The model under review builds one solid part; all positions refer to its coordinate system, in mm. A direction names the side the tool comes from. Coordinates: 2 decimals unless noted, no trailing zeros. Write each loop counter-clockwise with the first axis right and the second up, starting at its lowest first coordinate (ties: lowest second). Pieces come first, ordered by that corner, then holes.
1) Add section B-B, the plane z = 2.25. State the section outline as (x, y) points, then the cut area to 3 significant figures.
2) For line 1 (X direction, y = 0.2, z = -5.5); line 2 (X direction, y = 0.95, z = 2.75); line 3 (Y direction, x = 1.25, z = -3.75), list the stretches that pass through material, from the lowest coordinate up.
3) For P1, Ø0.9, axis at x = -0.5, y = -0.5, coming from the +Z side, flat-tipped, find the tip position at first contact; note if it passes through.
4) Machinability: for faces 3 (the cylindrical face through (-1.5, 0.07, 0)), 4 (the flat face through (-0.4, -0.4, -0.456)), which of the approach directions +Z, -Z, +X, -X, +Y, -Y give a long, thin tool a straight path to every point of the face, cutting with its end or side? Answer none if there is none.
5) Add section A-A, the plane y = 0.9. Give the number of separate pieces and of enclosed holes in the cut face, then the cut area to 3 significant figures.
6) Mouldability with a two-part tool opening along Z and no side actions: class faces 1 (the flat face through (-0.4, -0.4, -2.589)), 2 (the cylindrical face through (-1.5, 0.07, 2.14)) as released by +Z, released by -Z, zero draft, split by the parting line, or undercut.
from build123d import *

# Parameters (mm, degrees)
SKETCH1_R               = 1.5
BOSS_EXTRUDE1_DEPTH     = 4.8
SKETCH2_W               = 0.2
SKETCH2_H               = 3
CUT_EXTRUDE1_DEPTH      = 2.5
CUT_EXTRUDE1_DEPTH_BACK = 2.5
SKETCH3_R               = 0.375
BOSS_EXTRUDE2_DEPTH     = 6.5
SKETCH4_RX              = 0.5
SKETCH4_RY              = 0.25
BOSS_EXTRUDE3_DEPTH     = 1


with BuildPart() as part:
    # Sketch1 → Boss-Extrude1 (new body, symmetric)
    with BuildSketch(Plane.XY):
        Circle(SKETCH1_R)
    extrude(amount=BOSS_EXTRUDE1_DEPTH, both=True)

    # Sketch2 → Cut-Extrude1 (cut, two sides)
    with BuildSketch(Plane(origin=(0, 0, 0), x_dir=(0, 0, -1), z_dir=(1, 0, 0))) as cut_extrude1_sk:
        with Locations((-3.2, 0)):
            Rectangle(SKETCH2_W, SKETCH2_H)
        with Locations((-2.488888889, 0)):
            Rectangle(SKETCH2_W, SKETCH2_H)
        with Locations((-1.777777778, 0)):
            Rectangle(SKETCH2_W, SKETCH2_H)
        with Locations((-1.066666667, 0)):
            Rectangle(SKETCH2_W, SKETCH2_H)
        with Locations((-0.355555556, 0)):
            Rectangle(SKETCH2_W, SKETCH2_H)
        with Locations((0.355555556, 0)):
            Rectangle(SKETCH2_W, SKETCH2_H)
        with Locations((1.066666667, 0)):
            Rectangle(SKETCH2_W, SKETCH2_H)
        with Locations((1.777777778, 0)):
            Rectangle(SKETCH2_W, SKETCH2_H)
        with Locations((2.488888889, 0)):
            Rectangle(SKETCH2_W, SKETCH2_H)
        with Locations((3.2, 0)):
            Rectangle(SKETCH2_W, SKETCH2_H)
    extrude(amount=CUT_EXTRUDE1_DEPTH, mode=Mode.SUBTRACT)
    extrude(cut_extrude1_sk.sketch, amount=-CUT_EXTRUDE1_DEPTH_BACK, mode=Mode.SUBTRACT)

    # Sketch3 → Boss-Extrude2 (add, symmetric)
    with BuildSketch(Plane.XY):
        Circle(SKETCH3_R)
    extrude(amount=BOSS_EXTRUDE2_DEPTH, both=True)

    # Sketch4 → Boss-Extrude3 (add, symmetric)
    with BuildSketch(Plane(origin=(0, 0, 0), x_dir=(0, 0, -1), z_dir=(1, 0, 0))):
        with Locations((-5.5, 0.375)):
            Ellipse(SKETCH4_RX, SKETCH4_RY)
        with Locations(Location((5.5, 0.375), (0, 0, 180))):
            Ellipse(SKETCH4_RX, SKETCH4_RY)
    extrude(amount=BOSS_EXTRUDE3_DEPTH, both=True)


solid = part.part
Geometry results:
1. outline: circle Ø3 at (0, 0)
1. area: 7.07 mm2
2. line 1: x = -1 to 1
2. line 2: x = -1.16 to 1.16
2. line 3: y = -0.83 to 0.83
3. P1: stops at z = 6.5
4. face 3: +Z, -Z
4. face 4: none
5. separate pieces: 11
5. enclosed holes: 0
5. area: 18.2 mm2
6. face 1: undercut
6. face 2: zero draft
